Could you check a few things on this model? Use its own coordinates, in mm. Give positions to 0.01 mm unless a question says otherwise; leave off trailing zeros. Write each loop counter-clockwise with the first axis right and the second up, starting at its lowest first coordinate (ties: lowest second). Pieces come first, ordered by that corner, then holes. Notation, with made-up numbers: M 82,55 L 132,55 A23 ccw 132,76 Z; hole C -2.5,89.25 d8. An arc over 180 degrees is marked long. One line per item, written item: value.
```python
from build123d import *

# Parameters (mm, degrees)
SKETCH_R  = 3
PAD_DEPTH = 8


with BuildPart() as part:
    # Sketch → Pad (new body)
    with BuildSketch(Plane.YZ):
        Polygon((-5.277262, 5.001455), (44.722736, 4.987671), (44.719979, -5.012328), (-5.280019, -4.998545), align=None)
        Circle(SKETCH_R, mode=Mode.SUBTRACT)
    extrude(amount=PAD_DEPTH)


solid = part.part
```
1) I'm going to push a flat-ended pin straight in: pin 1 (1.5 mm diameter, centred on x = 7, y = 37.5, fed in from +Z). Where does the tip first touch, or does it pass through?
Outcome:
pin 1: stops at z = 4.99
2) If we section it at B-B, the plane x = 7.5: Write out the boundary of the cut face in (y, z).
Outcome:
outline: M -5.28,-5 L 44.72,-5.01 L 44.72,4.99 L -5.28,5 Z; hole C 0,0 d6
3) If we section it at A-A, the plane y = 0: Write out the boundary of the cut face in (x, z).
Outcome:
outline: M 0,-5 L 8,-5 L 8,-3 L 0,-3 Z; M 0,3 L 8,3 L 8,5 L 0,5 Z
4) If we section it at C-C, the plane z = 0: Write out the boundary of the cut face in (x, y), then the cut area to 3 significant figures.
Outcome:
outline: M 0,-5.28 L 8,-5.28 L 8,-3 L 0,-3 Z; M 0,3 L 8,3 L 8,44.72 L 0,44.72 Z
area: 352 mm^2
5) Please list where these lines run through material, in increasing order: L1, parallel to Z at x = 4, y = 0; L2, parallel to Z at x = 0.75, y = 4.5; L3, parallel to Y at x = 5.75, z = -2.5. Write a range as from..to.
Outcome:
L1: z = -5..-3, 3..5
L2: z = -5..5
L3: y = -5.28..-1.66, 1.66..44.72
6) We'd pull the mould along Z, two halves only. Please class faces 1 (the face through (4, -3, 0)), 2 (the face through (8, 20, 0)): pulls with the +Z half, pulls with the -Z half, needs draft (parallel to the pull), parting line crosses it, or undercut.
Outcome:
face 1: undercut
face 2: needs draft
